Design review of the part built by this model. Coordinates are the model's own, in mm. Face numbers are marked on the shaded views. A direction names the side the tool comes from. Give positions to 0.01 mm unless a question says otherwise; leave off trailing zeros. Write each loop counter-clockwise with the first axis right and the second up, starting at its lowest first coordinate (ties: lowest second). Pieces come first, ordered by that corner, then holes. Notation, with made-up numbers: (7, 6.25) -> (27, 6.25) arc R15 ccw to (27, 28.25) -> close; hole circle Ø6 at (70.5, 23.5). An arc over 180 degrees is marked (long way). Use CSV: the item, a comma, the result in double quotes.
```python
from build123d import *

# Parameters (mm, degrees)
CUT_EXTRUDE1_DEPTH          = 59.614042959
CIRPATTERN1_COUNT           = 6
SKETCH11_R                  = 5.953125
CUT_EXTRUDE3_DEPTH          = 59.614042959
F_4_40_TAPPED_HOLE2_D       = 2.2606
CUT_EXTRUDE4_DEPTH          = 59.614042959
F_1_2_13_TAPPED_HOLE1_D     = 10.71626
F_1_2_13_TAPPED_HOLE1_DEPTH = 28.829
F_1_2_13_TAPPED_HOLE1_TIP   = 3.219489309
CUT_EXTRUDE5_REACH          = 79.453
CUT_EXTRUDE5_END_RADIUS     = 19.05
SKETCH23_R                  = 5.953125
CUT_EXTRUDE6_REACH          = 59.777
SKETCH25_W                  = 87.993587341
SKETCH25_H                  = 27.156858223
CUT_EXTRUDE7_DEPTH          = 9.0805


with BuildPart() as part:
    # Sketch1 → Revolve1 (revolve)
    with BuildSketch(Plane.XY):
        Polygon((19.05, 0), (19.05, -31.75), (0, -31.75), (0, -38.1), (31.496, -38.1), (31.496, 0), (23.01875, 0), (22.225, -1.374815329), (21.43125, 0), align=None)
    revolve(axis=Axis((0, -582.039095303, 0), (0, 1, 0)))

    # Sketch2 → Cut-Extrude1 (cut, through all)
    with BuildSketch(Plane(origin=(0, 0, 0), x_dir=(1, 0, 0), z_dir=(0, 1, 0))):
        with BuildLine():
            Line((-10.432568811, 29.718), (10.432568811, 29.718))
            ThreePointArc((10.432568811, 29.718), (0, 31.496), (-10.432568811, 29.718))
        make_face()
    extrude(amount=-CUT_EXTRUDE1_DEPTH, mode=Mode.SUBTRACT)

    # Sketch5 → #8-32 Tapped Hole1 (revolve, cut)
    with BuildSketch(Plane(origin=(-13.49375, 0, -23.371860585), x_dir=(0, 0, 1), z_dir=(1, 0, 0))):
        Polygon((0, 0), (0, 18.208206461), (1.7272, 17.1704), (1.7272, 0), align=None)
    f_8_32_tapped_hole1 = revolve(axis=Axis((-13.49375, 6.35, -23.371860585), (0, -1, 0)), mode=Mode.SUBTRACT)

    # CirPattern1: #8-32 Tapped Hole1 ×6 about axis
    cirpattern1_axis = Axis((0, 0, 0), (0, 1, 0))
    for i in range(1, CIRPATTERN1_COUNT):
        add(f_8_32_tapped_hole1.rotate(cirpattern1_axis, i * 360 / CIRPATTERN1_COUNT), mode=Mode.SUBTRACT)

    # Sketch11 → Cut-Extrude3 (cut, through all)
    with BuildSketch(Plane.XZ.offset(38.1)):
        Circle(SKETCH11_R)
    extrude(amount=-CUT_EXTRUDE3_DEPTH, mode=Mode.SUBTRACT)

    # #4-40 Tapped Hole2 (through all)
    with Locations(Plane(origin=(0, -38.1, 0), x_dir=(-1, 0, 0), z_dir=(0, -1, 0))):
        with Locations((6.35, -6.35), (-6.35, -6.35), (-6.35, 6.35), (6.35, 6.35)):
            Hole(F_4_40_TAPPED_HOLE2_D / 2)

    # Sketch16 → Cut-Extrude4 (cut, through all)
    with BuildSketch(Plane.XZ.offset(38.1)):
        with BuildLine():
            Line((-9.873177996, 29.9085), (9.873177996, 29.9085))
            ThreePointArc((9.873177996, 29.9085), (0, 31.496), (-9.873177996, 29.9085))
        make_face()
    extrude(amount=-CUT_EXTRUDE4_DEPTH, mode=Mode.SUBTRACT)

    # 1/2-13 Tapped Hole1
    with Locations(Plane.XY.offset(29.9085)):
        with Locations((0, -25.4)):
            Hole(F_1_2_13_TAPPED_HOLE1_D / 2, depth=F_1_2_13_TAPPED_HOLE1_DEPTH)
            with Locations((0, 0, -(F_1_2_13_TAPPED_HOLE1_DEPTH + F_1_2_13_TAPPED_HOLE1_TIP / 2))):  # 118° drill point
                Cone(0, F_1_2_13_TAPPED_HOLE1_D / 2, F_1_2_13_TAPPED_HOLE1_TIP, mode=Mode.SUBTRACT)

    # Cut-Extrude5: up to this cylinder (the profile starts outside it)
    cut_extrude5_end = Plane(origin=(0, -22.225, 0), z_dir=(0, -1, 0)) * Cylinder(CUT_EXTRUDE5_END_RADIUS, 198.006, mode=Mode.PRIVATE)
    # Sketch23 → Cut-Extrude5 (cut, up to the surface)
    with BuildSketch(Plane(origin=(0, 0, -29.718), x_dir=(-1, 0, 0), z_dir=(0, 0, -1)), mode=Mode.PRIVATE) as cut_extrude5_sk1:
        with Locations((0, -22.225)):
            Circle(SKETCH23_R)
    cut_extrude5_tool1 = extrude(cut_extrude5_sk1.sketch, amount=-CUT_EXTRUDE5_REACH, mode=Mode.PRIVATE) - cut_extrude5_end
    add(cut_extrude5_tool1.solids().sort_by_distance((0, -22.225, -29.718))[0], mode=Mode.SUBTRACT)

    # Cut-Extrude6: up to this face of the body (flat: up to its plane)
    cut_extrude6_end = Plane(part.part.faces().sort_by_distance((-18.511184633, -31.75, 0))[0])
    # Sketch24 → Cut-Extrude6 (cut, up to the picked face)
    with BuildSketch(Plane(origin=(0, 0, 0), x_dir=(1, 0, 0), z_dir=(0, 1, 0)), mode=Mode.PRIVATE) as cut_extrude6_sk1:
        with BuildLine():
            Line((-7.9375, 19.05), (7.9375, 19.05))
            ThreePointArc((7.9375, 19.05), (11.305096045, 17.655096045), (12.7, 14.2875))
            Line((12.7, 14.2875), (12.7, 5.742929028))
            Line((12.7, 5.742929028), (-12.7, 5.742929028))
            Line((-12.7, 5.742929028), (-12.7, 14.2875))
            ThreePointArc((-12.7, 14.2875), (-11.305096045, 17.655096045), (-7.9375, 19.05))
        make_face()
    cut_extrude6_tool1 = split(extrude(cut_extrude6_sk1.sketch, amount=-CUT_EXTRUDE6_REACH, mode=Mode.PRIVATE), bisect_by=cut_extrude6_end, keep=Keep.BOTH, mode=Mode.PRIVATE)
    add(cut_extrude6_tool1.solids().sort_by(Axis((0, 0, -12.230696), (0, -1, 0)))[0], mode=Mode.SUBTRACT)

    # Sketch25 → Cut-Extrude7 (cut)
    with BuildSketch(Plane(origin=(0, 0, -29.718), x_dir=(-1, 0, 0), z_dir=(0, 0, -1))):
        with Locations((-3.719611081, -26.278429112)):
            Rectangle(SKETCH25_W, SKETCH25_H)
    extrude(amount=-CUT_EXTRUDE7_DEPTH, mode=Mode.SUBTRACT)


solid = part.part
```
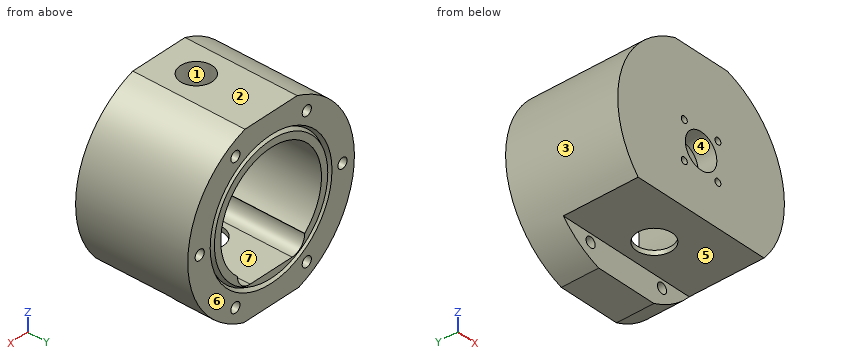
(1) Take a section at A-A (y = -34.5). Write out the cut boundary in (x, z).
Established:
outline,"(-23.79, -20.64) -> (23.79, -20.64) arc R31.5 ccw to (9.87, 29.91) -> (-9.87, 29.91) arc R31.5 ccw to start; hole circle Ø2.26 at (-6.35, -6.35); hole circle Ø2.26 at (-6.35, 6.35); hole circle Ø11.91 at (0, 0); hole circle Ø2.26 at (6.35, -6.35); hole circle Ø2.26 at (6.35, 6.35)"
(2) Tool access review of the marked faces 5, 6 and 7: name each direction out of +Z, -Z, +X, -X, +Y, -Y from which nothing blocks a thin tool from reaching the whole face with its end or side.
Established:
face 5,"-Z, +X, -X, -Y"
face 6,"+Z, -Z, +X, -X, +Y"
face 7,"+Y"
(3) Clearance check with flat-ended pins moving along their axes: pin 1 (19 mm diameter, centred on x = 7.5, z = 0, fed in from +Y); pin 2 (2 mm diameter, centred on x = 14, y = -24, fed in from -Z); pin 3 (8 mm diameter, centred on y = -10, z = 3, fed in from -X); pin 4 (10 mm diameter, centred on y = -5, z = -22.5, fed in from +X). State where each tip first meets the part, or that it passes through.
Established:
pin 1,"stops at y = -31.75"
pin 2,"stops at z = -20.64"
pin 3,"stops at x = -31.5"
pin 4,"stops at x = 26.19"
(4) Mouldability with a two-part tool opening along X and no side actions: class the marked faces 1, 2, 3 and 4 as +X half, -X half, draft (parallel to the pull), parting line (faces both ways), or undercut.
Established:
face 1,"undercut"
face 2,"draft"
face 3,"-X half"
face 4,"undercut"
(5) For line 1 along X through (y, z) = (-4, 0); line 2 along Z through (x, y) = (-6.35, -34); line 3 along Z through (x, y) = (0, -33.5), list the stretches that pass through material, from the lowest coordinate up. Write a range as [from, to].
Established:
line 1,"x = [-31.5, -28.71], [-25.26, -19.05], [19.05, 25.26], [28.71, 31.5]"
line 2,"z = [-20.64, -7.48], [-5.22, 5.22], [7.48, 29.91]"
line 3,"z = [-20.64, -5.95], [5.95, 29.91]"
(6) Take a section at B-B (y = -10.5). State how many separate pieces and enclosed holes the cut face has, then the cut area to 3 significant figures.
Established:
separate pieces,"1"
enclosed holes,"7"
area,"1,850 mm2"
